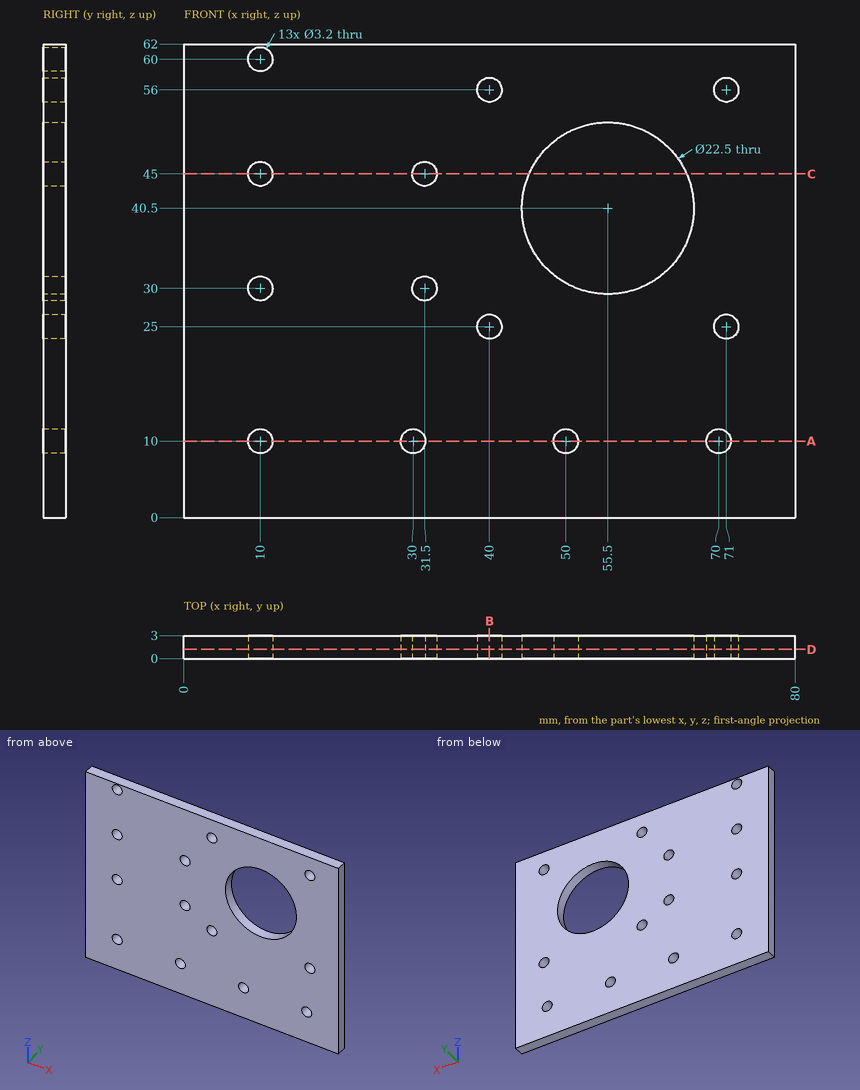
Here's the drawing with two shaded views (mm, measured from the low corner). I have some questions. Give positions to 0.01 mm unless a question says otherwise; leave off trailing zeros. Loops run counter-clockwise (first coordinate to the right, second up) from the corner with the lowest first, then second, coordinate; pieces in that order, holes last. Notation, with made-up numbers: (54.25, 0.25) - (87.25, 0.25) arc R26 ccw to (87.25, 36.25) - close; hole circle Ø5 at (39, 85.25). An arc over 180 degrees is marked (long way). Answer in a Markdown table with one row per item. Add a question column.
Q1. Please list where these lines run through material, in increasing order: L1, parallel to X at y = 1.2, z = 56; L2, parallel to X at y = 2.25, z = 45; L3, parallel to X at y = 2.1, z = 10. Write a range as from..to.
Q2. If we section it at A-A (z = 10): List the corners of the cut face in (x, y) for me, plus the area to 3 significant figures.
Q3. If we section it at B-B (x = 40): List the corners of the cut face in (y, z) for me, plus the area to 3 significant figures.
Q4. If we section it at D-D (y = 1.2): State how many separate pieces and enclosed holes the cut face has, plus the area to 3 significant figures.
Q5. If we section it at C-C (z = 45): List the corners of the cut face in (x, y) for me, plus the area to 3 significant figures.
The answers:
| question | item | result |
|---|---|---|
| 1 | L1 | x = 0..38.4, 41.6..69.4, 72.6..80 |
| 1 | L2 | x = 0..8.4, 11.6..29.9, 33.1..45.19, 65.81..80 |
| 1 | L3 | x = 0..8.4, 11.6..28.4, 31.6..48.4, 51.6..68.4, 71.6..80 |
| 2 | outline | (0, 0) - (8.4, 0) - (8.4, 3) - (0, 3) - close; (11.6, 0) - (28.4, 0) - (28.4, 3) - (11.6, 3) - close; (31.6, 0) - (48.4, 0) - (48.4, 3) - (31.6, 3) - close; (51.6, 0) - (68.4, 0) - (68.4, 3) - (51.6, 3) - close; (71.6, 0) - (80, 0) - (80, 3) - (71.6, 3) - close |
| 2 | area | 202 mm^2 |
| 3 | outline | (0, 0) - (3, 0) - (3, 23.4) - (0, 23.4) - close; (0, 26.6) - (3, 26.6) - (3, 54.4) - (0, 54.4) - close; (0, 57.6) - (3, 57.6) - (3, 62) - (0, 62) - close |
| 3 | area | 167 mm^2 |
| 4 | separate pieces | 1 |
| 4 | enclosed holes | 14 |
| 4 | area | 4,460 mm^2 |
| 5 | outline | (0, 0) - (8.4, 0) - (8.4, 3) - (0, 3) - close; (11.6, 0) - (29.9, 0) - (29.9, 3) - (11.6, 3) - close; (33.1, 0) - (45.19, 0) - (45.19, 3) - (33.1, 3) - close; (65.81, 0) - (80, 0) - (80, 3) - (65.81, 3) - close |
| 5 | area | 159 mm^2 |
